Build history of the part. All positions in model axes, mm. A direction names the side the tool comes from. Round coordinates to 2 decimals unless told otherwise and drop trailing zeros. Order: outer loops, then holes, each group sorted by start corner. A loop starts at its lowest first (then second) coordinate and runs counter-clockwise, first axis right, second up. Notation, with made-up numbers: M 78.5,-16.75 L 99.5,-16.75 A24 cw 99.5,-2.75 Z; hole C 27,-3.75 d8. An arc over 180 degrees is marked long. Use CSV: the item, a comma, the result in double quotes.
from build123d import *

# Parameters (mm, degrees)
SKETCH_W        = 56.771899
SKETCH_H        = 26
PAD_DEPTH       = 30
SKETCH001_W     = 15.2
SKETCH001_H     = 15.2
POCKET_DEPTH    = 30.001
SKETCH002_R     = 0.848528
SKETCH002_R_2   = 0.793369
POCKET001_DEPTH = 30.001
SKETCH003_W     = 2.8
SKETCH003_H     = 5.6
POCKET002_DEPTH = 6
SKETCH004_R     = 1.7
POCKET003_DEPTH = 7
SKETCH007_W     = 2.9
SKETCH007_H     = 5.8
POCKET004_DEPTH = 7
SKETCH008_W     = 6.5
SKETCH008_H     = 34.424917
POCKET005_DEPTH = 1
POCKET006_DEPTH = 2
SKETCH005_R     = 1.7
POCKET007_DEPTH = 17.001
FILLET_R        = 1
FILLET001_R     = 1
FILLET002_R     = 2


with BuildPart() as part:
    # Sketch → Pad (new body)
    with BuildSketch(Plane.XY):
        with Locations((-12.614051, 0)):
            Rectangle(SKETCH_W, SKETCH_H)
    extrude(amount=PAD_DEPTH)

    # Sketch001 → Pocket (cut, through all)
    with BuildSketch(Plane(origin=(0, 0, 0), x_dir=(1, 0, 0), z_dir=(0, 0, -1))):
        Rectangle(SKETCH001_W, SKETCH001_H)
        with BuildLine():
            ThreePointArc((-30.947343, -1), (-13.000044, -0.055902), (-30.941113, 1))
            Line((-42, 1), (-30.941113, 1))
            Line((-42, -1), (-42, 1))
            Line((-30.947343, -1), (-42, -1))
        make_face()
        with BuildLine():
            ThreePointArc((-14, 8.944272), (-24.9794, 11.617839), (-33.325879, 4))
            Line((-43, 4), (-33.325879, 4))
            Line((-43, 4), (-43, 14))
            Line((-43, 14), (-6, 14))
            Line((-6, 14), (-14, 8.944272))
        make_face()
        with BuildLine():
            Line((-6, -14), (-43, -14))
            Line((-43, -14), (-43, -5))
            Line((-32.944272, -5), (-43, -5))
            ThreePointArc((-32.944272, -5), (-24.483382, -11.789328), (-14, -9))
            Line((-14, -9), (-6, -14))
        make_face()
    extrude(amount=-POCKET_DEPTH, mode=Mode.SUBTRACT)

    # Sketch002 → Pocket001 (cut, through all)
    with BuildSketch(Plane(origin=(0, 0, 0), x_dir=(1, 0, 0), z_dir=(0, 0, -1))):
        with Locations((7.6, -7.6)):
            Circle(SKETCH002_R)
        with Locations((-7.6, -7.6)):
            Circle(SKETCH002_R_2)
        with Locations((-7.6, 7.6)):
            Circle(SKETCH002_R)
        with Locations((7.6, 7.6)):
            Circle(SKETCH002_R)
    extrude(amount=-POCKET001_DEPTH, mode=Mode.SUBTRACT)

    # Sketch003 → Pocket002 (cut)
    with BuildSketch(Plane(origin=(0, 0, 0), x_dir=(1, 0, 0), z_dir=(0, 0, -1))):
        with Locations((11.652548, 8.414147)):
            Rectangle(SKETCH003_W, SKETCH003_H)
        with Locations((11.645413, -0.129832)):
            Rectangle(SKETCH003_W, SKETCH003_H)
    extrude(amount=-POCKET002_DEPTH, mode=Mode.SUBTRACT)

    # Sketch004 → Pocket003 (cut)
    with BuildSketch(Plane.YZ.offset(15.771899)):
        with Locations((0, 3)):
            Circle(SKETCH004_R)
        with Locations((-8.3038, 3)):
            Circle(SKETCH004_R)
        with Locations((0, 27)):
            Circle(SKETCH004_R)
        with Locations((-8.3, 27)):
            Circle(SKETCH004_R)
    extrude(amount=-POCKET003_DEPTH, mode=Mode.SUBTRACT)

    # Sketch007 → Pocket004 (cut)
    with BuildSketch(Plane.XY.offset(30)):
        with Locations((11.597747, 0)):
            Rectangle(SKETCH007_W, SKETCH007_H)
        with Locations((11.580409, -7.890913)):
            Rectangle(SKETCH007_W, SKETCH007_H)
    extrude(amount=-POCKET004_DEPTH, mode=Mode.SUBTRACT)

    # Sketch008 → Pocket005 (cut)
    with BuildSketch(Plane.YZ.offset(15.771899)):
        with Locations((-3.946243, 14.212458)):
            Rectangle(SKETCH008_W, SKETCH008_H)
    extrude(amount=-POCKET005_DEPTH, mode=Mode.SUBTRACT)

    # Sketch006 → Pocket006 (cut)
    with BuildSketch(Plane(origin=(0, 5, 0), x_dir=(-1, 0, 0), z_dir=(0, 1, 0))):
        Polygon((39.8, 5.383419), (39.8, 8.616581), (37, 10.233162), (34.2, 8.616581), (34.2, 5.383419), (37, 3.766838), align=None)
    extrude(amount=-POCKET006_DEPTH, mode=Mode.SUBTRACT)

    # Sketch005 → Pocket007 (cut, through all)
    with BuildSketch(Plane.XZ.offset(4)):
        with Locations((-37, 7)):
            Circle(SKETCH005_R)
    extrude(amount=-POCKET007_DEPTH, mode=Mode.SUBTRACT)

    # Fillet
    fillet_edges = [part.edges().sort_by_distance(p)[0] for p in [
        (-41, -2.5, 0),
        (-41, 3, 0),
        (-41, 3, 30),
        (-41, -2.5, 30),
        (4.094768, -13, 0),
        (4.08595, 13, 0),
        (-37.162939, -4, 0),
        (-36.972136, 5, 0),
    ]]
    fillet(fillet_edges, radius=FILLET_R)

    # Fillet001
    fillet001_edges = [part.edges().sort_by_distance(p)[0] for p in [
        (4.094768, -13, 30),
        (4.08595, 13, 30),
    ]]
    fillet(fillet001_edges, radius=FILLET001_R)

    # Fillet002
    fillet002_edges = [part.edges().sort_by_distance(p)[0] for p in [
        (-13.000044, 0.055902, 30),
        (-13.000044, 0.055902, 0),
    ]]
    fillet(fillet002_edges, radius=FILLET002_R)


solid = part.part
(1) Two-plate mould, pull along Y, no slides. Class faces 4 (the face through (-35.7, 3, 5.6)), 5 (the face through (-38.42, 4.014, 9.414)), 6 (the face through (9.519, -0.221, 4.686)), 7 (the face through (8.2, -8.2, 14.8)): released by +Y, released by -Y, zero draft, split by the parting line, or undercut.
Answer block:
face 4,"released by +Y"
face 5,"zero draft"
face 6,"undercut"
face 7,"undercut"
(2) Tool access for faces 1 (the face through (-7.6, 0, 15)), 2 (the face through (9.46, -9.55, 28.15)), 3 (the face through (12, -2.67, 3)): list every direction of +Z, -Z, +X, -X, +Y, -Y with a clear straight run to the whole face (end or side of a thin tool).
Answer block:
face 1,"+Z, -Z"
face 2,"+X"
face 3,"-Z"
(3) Wall check: line 1 (Y direction, x = 12.5, z = 3.5); line 2 (Z direction, x = 13.95, y = -8.3); line 3 (Y direction, x = 14, z = 27). Give the ranges that are in metal, low to high. Write a range as from..to.
Answer block:
line 1,"y = -13..-11.21, -5.61..-2.67, 2.93..13"
line 2,"z = 0..1.3, 4.7..25.3, 28.7..30"
line 3,"y = -13..-10, -6.6..-1.7, 1.7..13"
(4) Drop flat-ended pins along their axis: pin 1 (1.7 mm diameter, centred on y = -9, z = 26.5, fed in from -X); pin 2 (1.7 mm diameter, centred on y = 0, z = 28, fed in from -X); pin 3 (4 mm diameter, centred on x = -37, z = 7, fed in from -Y). Give the stop position or say it passes through.
Answer block:
pin 1,"stops at x = -30.81"
pin 2,"stops at x = -13.04"
pin 3,"stops at y = -4"
(5) Cut at B-B, the plane y = 0. Count the separate pieces of the cut face and the enclosed holes in it, and give its area (3 significant figures).
Answer block:
separate pieces,"4"
enclosed holes,"0"
area,"340 mm²"
(6) Cut at A-A, the plane z = 15.5. Give the cut face in (x, y), and give its area (3 significant figures).
Answer block:
outline,"M -41,-4 L -33.33,-4 A12.02 ccw -14,-8.94 L -7.58,-13 L 15.77,-13 L 15.77,-7.2 L 14.77,-7.2 L 14.77,-0.7 L 15.77,-0.7 L 15.77,13 L -7.6,13 L -14,9 A12.02 ccw -32.94,5 L -41,5 L -41,1 L -30.95,1 A9 cw long -30.94,-1 L -41,-1 Z; hole M -7.6,-6.75 A0.85 ccw long -6.75,-7.6 L 6.75,-7.6 A0.85 ccw long 7.6,-6.75 L 7.6,6.75 A0.85 ccw long 6.75,7.6 L -6.81,7.6 A0.79 ccw long -7.6,6.81 Z"
area,"699 mm²"
